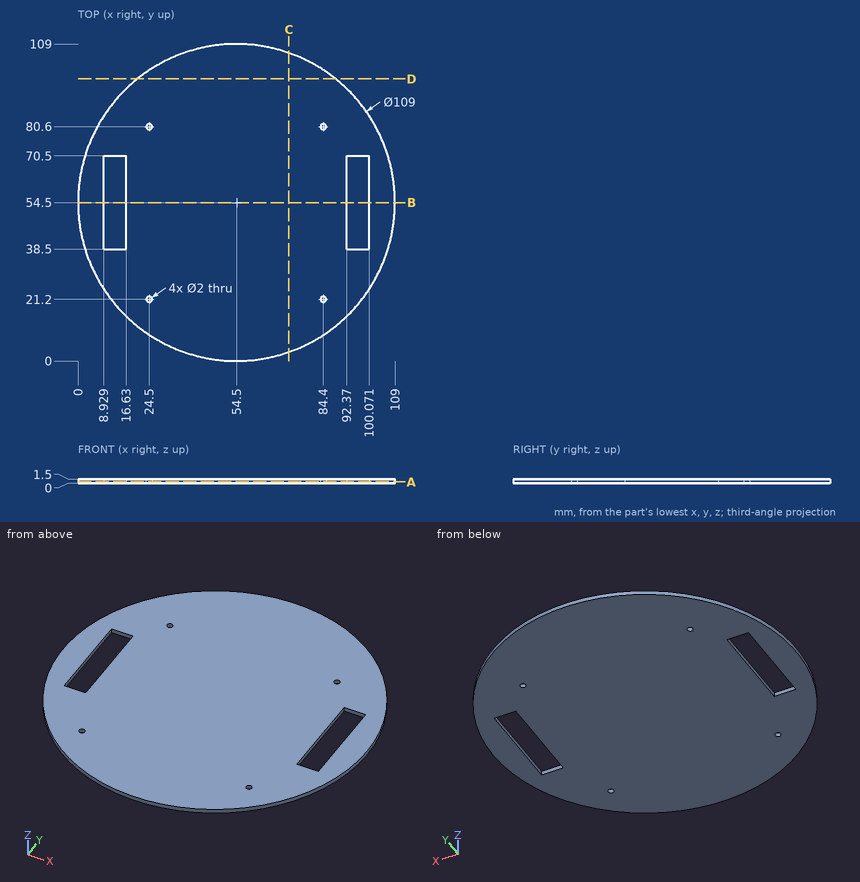
Input: dimensioned drawing with shaded views. Units: mm. Origin: part minimum x, y, z. Give positions to 0.01 mm unless a question says otherwise; leave off trailing zeros. Loops run counter-clockwise (first coordinate to the right, second up) from the corner with the lowest first, then second, coordinate; pieces in that order, holes last. Notation, with made-up numbers: (13.5, -2) -> (50.5, -2) arc R21 ccw to (50.5, 7) -> close; hole circle Ø2 at (51.25, 34.25). An arc over 180 degrees is marked (long way). Use a Markdown table: item, result.
Q1. Section query C-C, the plane x = 72.5. Return the cut outline in (y, z).
Entries:
| item | result |
|---|---|
| outline | (3.06, 0) -> (105.94, 0) -> (105.94, 1.5) -> (3.06, 1.5) -> close |
Q2. First-contact query: P1, Ø0.8, axis at x = 12, z = 0.5, coming from the +Y side. Flat tip, straight axial feed; report the tip coordinate or a pass-through.
Entries:
| item | result |
|---|---|
| P1 | stops at y = 89.11 |
Q3. Section query D-D, the plane y = 97. Return the cut outline in (x, z), plus the area to 3 significant figures.
Entries:
| item | result |
|---|---|
| outline | (20.38, 0) -> (88.62, 0) -> (88.62, 1.5) -> (20.38, 1.5) -> close |
| area | 102 mm² |
Q4. Section query B-B, the plane y = 54.5. Return the cut outline in (x, z).
Entries:
| item | result |
|---|---|
| outline | (0, 0) -> (8.93, 0) -> (8.93, 1.5) -> (0, 1.5) -> close; (16.63, 0) -> (92.37, 0) -> (92.37, 1.5) -> (16.63, 1.5) -> close; (100.07, 0) -> (109, 0) -> (109, 1.5) -> (100.07, 1.5) -> close |
Q5. Ray query, probe 1 along X at (y, z) = (47, 0.35); probe 2 along Y at (x, z) = (85, 1.15) (1 decimal); probe 3 along X at (y, z) = (60, 0.65). Return the intervals inside material, ascending. Write a range as from..to.
Entries:
| item | result |
|---|---|
| probe 1 | x = 0.52..8.93, 16.63..92.37, 100.07..108.48 |
| probe 2 | y = 9.3..20.4, 22..79.8, 81.4..99.7 |
| probe 3 | x = 0.28..8.93, 16.63..92.37, 100.07..108.72 |
Q6. Section query A-A, the plane z = 0.5. Return the cut outline in (x, y).
Entries:
| item | result |
|---|---|
| outline | circle Ø109 at (54.5, 54.5); hole (8.93, 38.5) -> (16.63, 38.5) -> (16.63, 70.5) -> (8.93, 70.5) -> close; hole circle Ø2 at (24.5, 21.2); hole circle Ø2 at (24.5, 80.6); hole circle Ø2 at (84.4, 21.2); hole circle Ø2 at (84.4, 80.6); hole (92.37, 38.5) -> (100.07, 38.5) -> (100.07, 70.5) -> (92.37, 70.5) -> close |
